The listing builds one solid part. Answer for the finished solid, in the listing's coordinates (mm). Face numbers are marked on the shaded views. A direction names the side the tool comes from. Round coordinates to 2 decimals unless told otherwise and drop trailing zeros. Write each loop counter-clockwise with the first axis right and the second up, starting at its lowest first coordinate (ties: lowest second). Pieces come first, ordered by that corner, then holes.
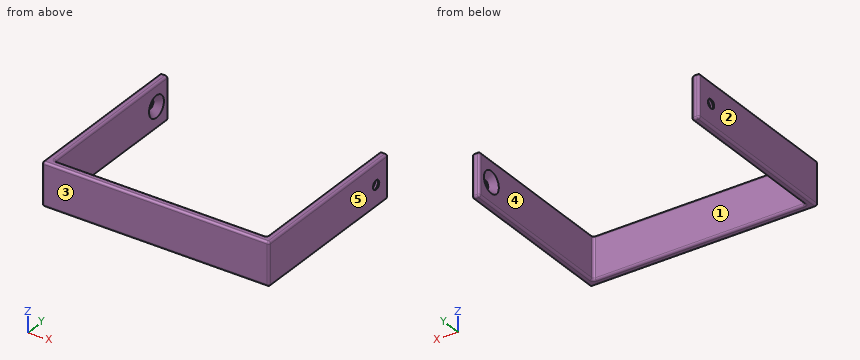
from build123d import *

# Parameters (mm, degrees)
SKETCH1_W           = 20
SKETCH1_H           = 80
BOSS_EXTRUDE1_DEPTH = 105.6
CUT_EXTRUDE1_REACH  = 135.983
SKETCH2_W           = 98.6
SKETCH2_H           = 76.5
FILLET1_R           = 1


with BuildPart() as part:
    # Sketch1 → Boss-Extrude1 (new body)
    with BuildSketch(Plane(origin=(0, 0, 0), x_dir=(0, 0, -1), z_dir=(1, 0, 0))):
        with Locations((0, 40)):
            Rectangle(SKETCH1_W, SKETCH1_H)
    extrude(amount=-BOSS_EXTRUDE1_DEPTH)

    # Sketch2 → Cut-Extrude1 (cut, up to next)
    with BuildSketch(Plane(origin=(0, 0, -10), x_dir=(-1, 0, 0), z_dir=(0, 0, -1)), mode=Mode.PRIVATE) as cut_extrude1_sk1:
        with Locations((52.8, 41.75)):
            Rectangle(SKETCH2_W, SKETCH2_H)
    cut_extrude1_tool1 = extrude(cut_extrude1_sk1.sketch, amount=-CUT_EXTRUDE1_REACH, mode=Mode.PRIVATE) & part.part
    add(cut_extrude1_tool1.solids().sort_by_distance((-52.8, 41.75, -10))[0], mode=Mode.SUBTRACT)

    # Sketch4 → M5 Tapped Hole2 (revolve, cut)
    with BuildSketch(Plane(origin=(-102.1, 72, 0), x_dir=(0, 0, -1), z_dir=(0, 1, 0))):
        Polygon((0, 0), (0, 3.5), (2.1, 3.5), (2.1, 2.9), (5, 0), align=None)
    revolve(axis=Axis((-95.75, 72, 0), (-1, 0, 0)), mode=Mode.SUBTRACT)

    # Sketch15 → M5 Tapped Hole1 (revolve, cut)
    with BuildSketch(Plane(origin=(-3.5, 72, 0), x_dir=(0, 0, 1), z_dir=(0, 1, 0))):
        Polygon((0, 0), (0, 3.5), (2.1, 3.5), (2.1, 2.9), (5, 0), align=None)
    revolve(axis=Axis((-9.85, 72, 0), (1, 0, 0)), mode=Mode.SUBTRACT)

    # Fillet1
    fillet1_edges = [part.edges().sort_by_distance(p)[0] for p in [
        (-105.6, 40, -10),
        (-105.6, 80, 0),
        (-1.75, 80, -10),
        (-1.75, 80, 10),
        (-3.5, 41.75, 10),
        (-3.5, 3.5, 0),
        (-3.5, 80, 0),
        (-102.1, 41.75, 10),
        (-102.1, 80, 0),
        (-52.8, 3.5, 10),
        (-102.1, 3.5, 0),
        (-3.5, 41.75, -10),
        (-52.8, 3.5, -10),
        (-102.1, 41.75, -10),
        (-105.6, 40, 10),
        (0, 80, 0),
        (0, 40, -10),
        (0, 0, 0),
        (0, 40, 10),
        (-105.6, 0, 0),
        (-103.85, 80, 10),
        (-103.85, 80, -10),
        (-52.8, 0, -10),
        (-52.8, 0, 10),
    ]]
    fillet(fillet1_edges, radius=FILLET1_R)


solid = part.part
1. Given pin 1 (9 mm diameter, centred on x = -71.5, z = 2, fed in from +Y), flat-ended and moving along its own axis, determine where the tip first touches the part or whether it passes through.
Geometry says:
pin 1: stops at y = 3.5
2. Section C-C on x = -65 is taken. Determine the outline of the cut face in (y, z).
Geometry says:
outline: (0, -9) arc R1 ccw to (1, -10) - (2.5, -10) arc R1 ccw to (3.5, -9) - (3.5, 9) arc R1 ccw to (2.5, 10) - (1, 10) arc R1 ccw to (0, 9) - close
3. Section B-B on z = 0 is taken. Determine the outline of the cut face in (x, y).
Geometry says:
outline: (-105.6, 1) arc R1 ccw to (-104.6, 0) - (-1, 0) arc R1 ccw to (0, 1) - (0, 69.9) - (-0.6, 69.9) - (-3.5, 67) - (-3.5, 4.5) arc R1 cw to (-4.5, 3.5) - (-101.1, 3.5) arc R1 cw to (-102.1, 4.5) - (-102.1, 67) - (-105, 69.9) - (-105.6, 69.9) - close; (-105.6, 74.1) - (-105, 74.1) - (-102.1, 77) - (-102.1, 79) arc R1 ccw to (-103.1, 80) - (-104.6, 80) arc R1 ccw to (-105.6, 79) - close; (-3.5, 77) - (-0.6, 74.1) - (0, 74.1) - (0, 79) arc R1 ccw to (-1, 80) - (-2.5, 80) arc R1 ccw to (-3.5, 79) - close
4. Straight lines are drawn through the part: line 1 along X through (y, z) = (64, 6.25); line 2 along Y through (x, z) = (-35, -2.25); line 3 along Z through (x, y) = (-0.2, 72). For each, find the intervals that lie inside material, in ascending order.
Geometry says:
line 1: x = -105.6 to -102.1, -3.5 to 0
line 2: y = 0 to 3.5
line 3: z = -9.6 to -2.1, 2.1 to 9.6
5. A tool of negligible diameter and unlimited length cuts with its end or side. For the marked faces 1 and 2, from which of +Z, -Z, +X, -X, +Y, -Y can it reach the whole face along a straight path? Write none if from no direction.
Geometry says:
face 1: +Z, -Z, +Y
face 2: +Z, -Z, -X, +Y, -Y
6. Section D-D on y = 72 is taken. Determine the outline of the cut face in (x, z), plus the area to 3 significant figures.
Geometry says:
outline: (-105.6, -9) arc R1 ccw to (-104.6, -10) - (-103.1, -10) arc R1 ccw to (-102.1, -9) - (-102.1, -5) - (-105, -2.1) - (-105.6, -2.1) - close; (-105.6, 2.1) - (-105, 2.1) - (-102.1, 5) - (-102.1, 9) arc R1 ccw to (-103.1, 10) - (-104.6, 10) arc R1 ccw to (-105.6, 9) - close; (-3.5, -9) arc R1 ccw to (-2.5, -10) - (-1, -10) arc R1 ccw to (0, -9) - (0, -2.1) - (-0.6, -2.1) - (-3.5, -5) - close; (-3.5, 5) - (-0.6, 2.1) - (0, 2.1) - (0, 9) arc R1 ccw to (-1, 10) - (-2.5, 10) arc R1 ccw to (-3.5, 9) - close
area: 92.1 mm2
7. Section A-A on y = 60 is taken. Determine the outline of the cut face in (x, z).
Geometry says:
outline: (-105.6, -9) arc R1 ccw to (-104.6, -10) - (-103.1, -10) arc R1 ccw to (-102.1, -9) - (-102.1, 9) arc R1 ccw to (-103.1, 10) - (-104.6, 10) arc R1 ccw to (-105.6, 9) - close; (-3.5, -9) arc R1 ccw to (-2.5, -10) - (-1, -10) arc R1 ccw to (0, -9) - (0, 9) arc R1 ccw to (-1, 10) - (-2.5, 10) arc R1 ccw to (-3.5, 9) - close
8. For a pull along X with two mould halves and no side action, classify the marked faces 3, 4 and 5 as released by +X, released by -X, zero draft, split by the parting line, or undercut.
Geometry says:
face 3: zero draft
face 4: undercut
face 5: released by +X
